Read the model definition and answer for the solid it produces. Units are mm, in the model's axes. A direction names the side the tool comes from. Coordinates: 2 decimals unless noted, no trailing zeros. Loops run counter-clockwise (first coordinate to the right, second up) from the corner with the lowest first, then second, coordinate; pieces in that order, holes last. Notation, with made-up numbers: (-26.5, 23) -> (-19.5, 23) arc R26 cw to (-19.5, 58) -> close; hole circle Ø6 at (22.25, -18). An arc over 180 degrees is marked (long way). Answer in a Markdown table with one row per item.
```python
from build123d import *

# Parameters (mm, degrees)
BOSS_EXTRUDE1_DEPTH = 60
CUT_EXTRUDE2_REACH  = 19.614
SKETCH3_R           = 1.9
SKETCH4_R           = 4.4
CUT_EXTRUDE3_DEPTH  = 10


with BuildPart() as part:
    # Sketch1 → Boss-Extrude1 (new body)
    with BuildSketch(Plane(origin=(0, 0, 0), x_dir=(1, 0, 0), z_dir=(0, 1, 0))):
        with BuildLine():
            Line((0, 10), (-10, 10))
            ThreePointArc((-10, 10), (-19.384585633, 3.453918427), (-16.48271865, -7.6140895))
            Line((-16.48271865, -7.6140895), (-12.924300248, -4.055671098))
            ThreePointArc((-12.924300248, -4.055671098), (-13.535533906, -3.535533906), (-14.055671098, -2.924300248))
            Line((-14.055671098, -2.924300248), (-16.194184337, -5.062813487))
            ThreePointArc((-16.194184337, -5.062813487), (-18, 0), (-16.194184337, 5.062813487))
            Line((-16.194184337, 5.062813487), (-14.055671098, 2.924300248))
            ThreePointArc((-14.055671098, 2.924300248), (-13.535533906, 3.535533906), (-12.924300248, 4.055671098))
            Line((-12.924300248, 4.055671098), (-15.062813487, 6.194184337))
            ThreePointArc((-15.062813487, 6.194184337), (-10, 8), (-4.937186513, 6.194184337))
            Line((-4.937186513, 6.194184337), (-7.075699752, 4.055671098))
            ThreePointArc((-7.075699752, 4.055671098), (-6.464466094, 3.535533906), (-5.944328902, 2.924300248))
            Line((-5.944328902, 2.924300248), (-3.805815663, 5.062813487))
            ThreePointArc((-3.805815663, 5.062813487), (-2, 0), (-3.805815663, -5.062813487))
            Line((-3.805815663, -5.062813487), (-5.944328902, -2.924300248))
            ThreePointArc((-5.944328902, -2.924300248), (-6.464466094, -3.535533906), (-7.075699752, -4.055671098))
            Line((-7.075699752, -4.055671098), (-3.51728135, -7.6140895))
            Line((-3.51728135, -7.6140895), (15, -7.6140895))
            Line((15, -7.6140895), (15, 1.19295525))
            Line((15, 1.19295525), (15, 10))
            Line((15, 10), (0, 10))
        make_face()
    extrude(amount=BOSS_EXTRUDE1_DEPTH)

    # Sketch3 → Cut-Extrude2 (cut, up to next)
    with BuildSketch(Plane(origin=(0, 0, -10), x_dir=(-1, 0, 0), z_dir=(0, 0, -1)), mode=Mode.PRIVATE) as cut_extrude2_sk1:
        with Locations((-5, 42.5)):
            Circle(SKETCH3_R)
    cut_extrude2_tool1 = extrude(cut_extrude2_sk1.sketch, amount=-CUT_EXTRUDE2_REACH, mode=Mode.PRIVATE) & part.part
    add(cut_extrude2_tool1.solids().sort_by_distance((5, 42.5, -10))[0], mode=Mode.SUBTRACT)
    # Sketch3 → Cut-Extrude2 (cut, up to next)
    with BuildSketch(Plane(origin=(0, 0, -10), x_dir=(-1, 0, 0), z_dir=(0, 0, -1)), mode=Mode.PRIVATE) as cut_extrude2_sk2:
        with Locations((-5, 17.5)):
            Circle(SKETCH3_R)
    cut_extrude2_tool2 = extrude(cut_extrude2_sk2.sketch, amount=-CUT_EXTRUDE2_REACH, mode=Mode.PRIVATE) & part.part
    add(cut_extrude2_tool2.solids().sort_by_distance((5, 17.5, -10))[0], mode=Mode.SUBTRACT)

    # Sketch4 → Cut-Extrude3 (cut)
    with BuildSketch(Plane(origin=(15, 0, 0), x_dir=(0, 0, -1), z_dir=(1, 0, 0))):
        with Locations((1.19295525, 7.5)):
            Circle(SKETCH4_R)
        with Locations((1.19295525, 52.5)):
            Circle(SKETCH4_R)
    extrude(amount=-CUT_EXTRUDE3_DEPTH, mode=Mode.SUBTRACT)


solid = part.part
```
1. The mould has two halves that part along X. Classify faces 1 (the cylindrical face through (-2, 30, 0)), 2 (the flat face through (1, 60, -1)), 3 (the flat face through (15, 30, -1)), 4 (the flat face through (-15.14, 29.58, -4.01)): pulls with the +X half, pulls with the -X half, needs draft (parallel to the pull), parting line crosses it, or undercut.
A:
| item | result |
|---|---|
| face 1 | undercut |
| face 2 | needs draft |
| face 3 | pulls with the +X half |
| face 4 | undercut |
2. A cutting plane is placed at C-C on y = 7.5. Give the vertices of the cut face in (x, z), and give its area (3 significant figures).
A:
| item | result |
|---|---|
| outline | (-16.48, 7.61) arc R10 ccw to (-10, -10) -> (15, -10) -> (15, -5.59) -> (5, -5.59) -> (5, 3.21) -> (15, 3.21) -> (15, 7.61) -> (-3.52, 7.61) -> (-7.08, 4.06) arc R5 cw to (-5.94, 2.92) -> (-3.81, 5.06) arc R8 cw to (-3.81, -5.06) -> (-5.94, -2.92) arc R5 cw to (-7.08, -4.06) -> (-4.94, -6.19) arc R8 cw to (-15.06, -6.19) -> (-12.92, -4.06) arc R5 cw to (-14.06, -2.92) -> (-16.19, -5.06) arc R8 cw to (-16.19, 5.06) -> (-14.06, 2.92) arc R5 cw to (-12.92, 4.06) -> close |
| area | 313 mm2 |
3. Given pin 1 Ø2.5 at (y, z) = (8, -0.5) entering from +X, flat-ended and moving along its own axis, determine where the tip first touches the part or whether it passes through.
A:
| item | result |
|---|---|
| pin 1 | stops at x = 5 |
4. A cutting plane is placed at D-D on x = 4. Give the vertices of the cut face in (y, z).
A:
| item | result |
|---|---|
| outline | (0, -10) -> (15.88, -10) -> (15.88, 7.61) -> (0, 7.61) -> close; (19.12, -10) -> (40.88, -10) -> (40.88, 7.61) -> (19.12, 7.61) -> close; (44.12, -10) -> (60, -10) -> (60, 7.61) -> (44.12, 7.61) -> close |
5. A cutting plane is placed at B-B on y = 42.5. Give the vertices of the cut face in (x, z).
A:
| item | result |
|---|---|
| outline | (-16.48, 7.61) arc R10 ccw to (-10, -10) -> (3.1, -10) -> (3.1, 7.61) -> (-3.52, 7.61) -> (-7.08, 4.06) arc R5 cw to (-5.94, 2.92) -> (-3.81, 5.06) arc R8 cw to (-3.81, -5.06) -> (-5.94, -2.92) arc R5 cw to (-7.08, -4.06) -> (-4.94, -6.19) arc R8 cw to (-15.06, -6.19) -> (-12.92, -4.06) arc R5 cw to (-14.06, -2.92) -> (-16.19, -5.06) arc R8 cw to (-16.19, 5.06) -> (-14.06, 2.92) arc R5 cw to (-12.92, 4.06) -> close; (6.9, -10) -> (15, -10) -> (15, 7.61) -> (6.9, 7.61) -> close |
6. Find the intervals of material crossed by probe 1 along Y at (x, z) = (8.5, -1.25); probe 2 along X at (y, z) = (22.5, -3.5); probe 3 along X at (y, z) = (48, -4), in increasing order.
A:
| item | result |
|---|---|
| probe 1 | y = 0 to 3.1, 11.9 to 48.1, 56.9 to 60 |
| probe 2 | x = -19.37 to -17.19, -14.63 to -13.57, -6.43 to -5.37, -2.81 to 15 |
| probe 3 | x = -19.17 to -16.93, -15.13 to -13, -7 to -4.87, -3.07 to 15 |
7. A cutting plane is placed at A-A on z = -0.5. Give the vertices of the cut face in (x, y), and give its area (3 significant figures).
A:
| item | result |
|---|---|
| outline | (-19.99, 0) -> (-17.98, 0) -> (-17.98, 60) -> (-19.99, 60) -> close; (-2.02, 0) -> (15, 0) -> (15, 3.15) -> (5, 3.15) -> (5, 11.85) -> (15, 11.85) -> (15, 48.15) -> (5, 48.15) -> (5, 56.85) -> (15, 56.85) -> (15, 60) -> (-2.02, 60) -> close; hole circle Ø3.8 at (5, 17.5); hole circle Ø3.8 at (5, 42.5) |
| area | 945 mm2 |
8. A tool of negligible diameter and unlimited length cuts with its end or side. For faces 5 (the flat face through (6, 30, 7.614)), 6 (the cylindrical face through (-6.46, 29.58, 3.53)), 7 (the flat face through (-5.32, 29.58, 5.81)), 8 (the cylindrical face through (10.07, 3.205, -0.239)), from which of +Z, -Z, +X, -X, +Y, -Y can it reach the whole face along a straight path? Write none if from no direction.
A:
| item | result |
|---|---|
| face 5 | +Z, +X, -X, +Y, -Y |
| face 6 | +Y, -Y |
| face 7 | +Z, +Y, -Y |
| face 8 | +X |
